Drawing for the job (mm, zero at the part's lowest x, y, z). A direction names the side the tool comes from. Give positions to 0.01 mm unless a question says otherwise; leave off trailing zeros. Loops run counter-clockwise (first coordinate to the right, second up) from the corner with the lowest first, then second, coordinate; pieces in that order, holes last. Notation, with made-up numbers: (77, 67) -> (112, 67) arc R20 ccw to (112, 101) -> close; hole circle Ø1 at (-31, 10.25). An arc over 180 degrees is marked (long way). Answer in a Markdown table with one row per item. Add a question column.
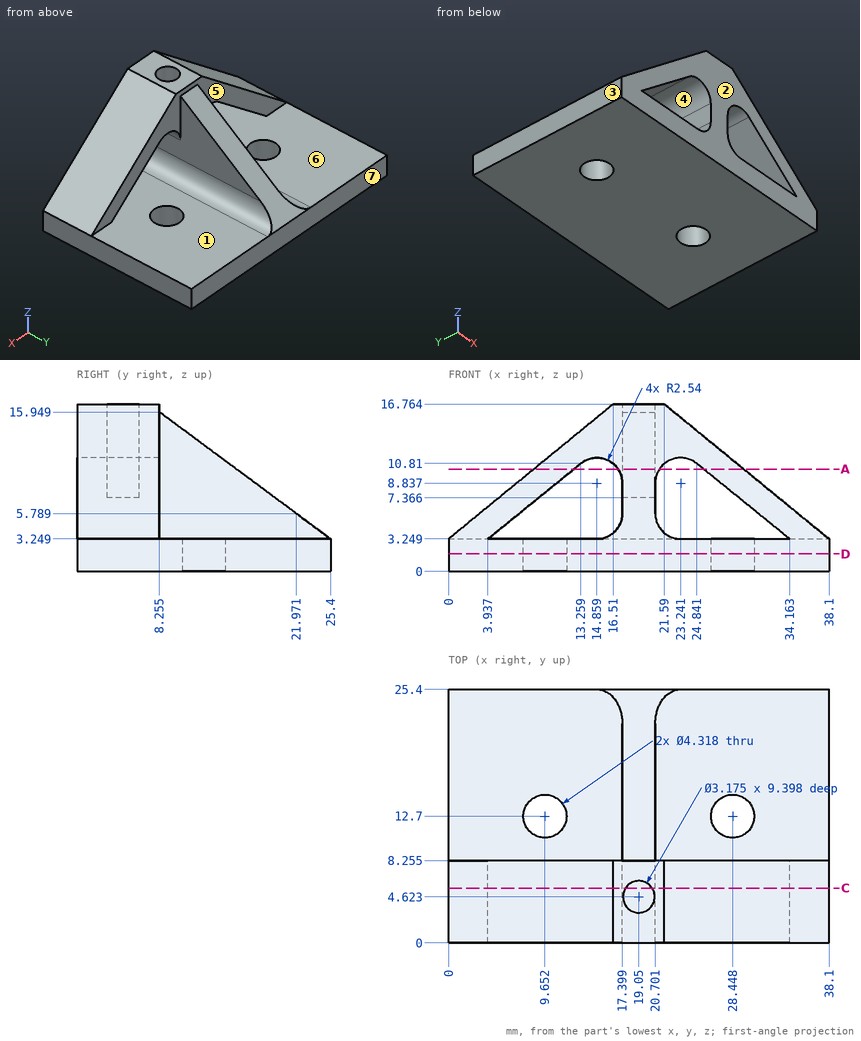
(1) Saw through at D-D, the plane z = 1.75. List the corners of the cut face in (x, y).
(2) 3-axis set-ups, long thin cutter, end or side, ignore diameter. For the marked faces 4, 5, 6 and 7: which of +Z, -Z, +X, -X, +Y, -Y reach the whole face in a straight line?
(3) Wall check: line 1 along Y through (x, z) = (27, 11.5) (1 decimal); line 2 along Z through (x, y) = (8, 14.5); line 3 along Z through (x, y) = (16, 4.25) (1 decimal). Give the ranges that are in metal, low to high. Write a range as from..to.
(4) Flat gauge pins, fed straight in: pin 1 Ø7 at (x, y) = (9.652, 12.7) entering from -Z; pin 2 Ø1 at (x, y) = (14.5, 17.5) entering from +Z; pin 3 Ø4 at (x, z) = (24.5, 9) entering from +Y (3 decimals); pin 4 Ø1 at (x, y) = (18.5, 5) entering from +Z. Where does each tip first touch, or does it go through?
(5) Saw through at A-A, the plane z = 10.25. State how many separate pieces and enclosed holes the cut face has, then the cut area to 3 significant figures.
(6) Saw through at C-C, the plane y = 5.5. List the corners of the cut face in (x, z).
(7) Two-plate mould, pull along X, no slides. Class the marked faces 1, 2 and 3: released by +X, released by -X, zero draft, split by the parting line, or undercut.
Worked answers:
| question | item | result |
|---|---|---|
| 1 | outline | (0, 0) -> (38.1, 0) -> (38.1, 25.4) -> (0, 25.4) -> close; hole circle Ø4.32 at (9.65, 12.7); hole circle Ø4.32 at (28.45, 12.7) |
| 2 | face 4 | +Y, -Y |
| 2 | face 5 | +Z, +Y |
| 2 | face 6 | +Y |
| 2 | face 7 | +Z, -Z, +X, -X, +Y |
| 3 | line 1 | 0..8.3 |
| 3 | line 2 | 0..3.25 |
| 3 | line 3 | 0..3.5, 11.1..16.3 |
| 4 | pin 1 | z = 0 |
| 4 | pin 2 | z = 3.25 |
| 4 | pin 3 | y = 8.255 |
| 4 | pin 4 | z = 7.37 |
| 5 | separate pieces | 3 |
| 5 | enclosed holes | 1 |
| 5 | area | 118 mm^2 |
| 6 | outline | (0, 0) -> (38.1, 0) -> (38.1, 3.25) -> (21.59, 16.76) -> (20.37, 16.76) -> (20.37, 7.37) -> (17.73, 7.37) -> (17.73, 16.76) -> (16.51, 16.76) -> (0, 3.25) -> close; hole (3.94, 3.25) -> (14.86, 3.25) arc R2.54 ccw to (17.4, 5.79) -> (17.4, 8.84) arc R2.54 ccw to (13.26, 10.81) -> close; hole (20.7, 5.79) arc R2.54 ccw to (23.24, 3.25) -> (34.16, 3.25) -> (24.84, 10.81) arc R2.54 ccw to (20.7, 8.84) -> close |
| 7 | face 1 | undercut |
| 7 | face 2 | zero draft |
| 7 | face 3 | released by -X |
